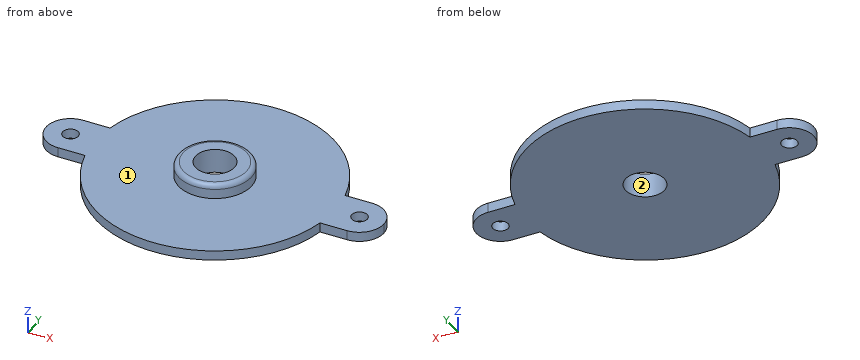
```python
from build123d import *

# Parameters (mm, degrees)
F0_R     = 1.6
F0_R_2   = 4
F1_DEPTH = 2
F2_R     = 7.5
F2_R_2   = 4
F3_DEPTH = 3
F4_R     = 1


with BuildPart() as f1:
    # F0 (on Top) → F1 (new body)
    with BuildSketch(Plane.XY):
        with BuildLine():
            ThreePointArc((-29.5, -5), (-25.964466, -3.535534), (-24.5, 0))
            ThreePointArc((-24.5, 0), (-25.964466, 3.535534), (-29.5, 5))
            ThreePointArc((-29.5, 5), (-34.5, 0), (-29.5, -5))
        make_face()
        with Locations((-29.5, 0)):
            Circle(F0_R, mode=Mode.SUBTRACT)
        with BuildLine():
            ThreePointArc((-29.5, 5), (-25.964466, 3.535534), (-24.5, 0))
            ThreePointArc((-24.5, 0), (-24.370752, 2.513259), (-23.98437, 5))
            Line((-23.98437, 5), (-29.5, 5))
        make_face()
        with BuildLine():
            ThreePointArc((-23.98437, -5), (-24.370752, -2.513259), (-24.5, 0))
            ThreePointArc((-24.5, 0), (-25.964466, -3.535534), (-29.5, -5))
            Line((-29.5, -5), (-23.98437, -5))
        make_face()
        with BuildLine():
            ThreePointArc((-23.98437, 5), (-24.370752, 2.513259), (-24.5, 0))
            ThreePointArc((-24.5, 0), (-24.370752, -2.513259), (-23.98437, -5))
            ThreePointArc((-23.98437, -5), (0, -24.5), (23.98437, -5))
            ThreePointArc((23.98437, -5), (24.370752, -2.513259), (24.5, 0))
            ThreePointArc((24.5, 0), (24.370752, 2.513259), (23.98437, 5))
            ThreePointArc((23.98437, 5), (0, 24.5), (-23.98437, 5))
        make_face()
        Circle(F0_R_2, mode=Mode.SUBTRACT)
        with BuildLine():
            ThreePointArc((29.5, 5), (25.964466, 3.535534), (24.5, 0))
            ThreePointArc((24.5, 0), (25.964466, -3.535534), (29.5, -5))
            ThreePointArc((29.5, -5), (33.035534, -3.535534), (34.5, 0))
            ThreePointArc((34.5, 0), (33.035534, 3.535534), (29.5, 5))
        make_face()
        with Locations((29.5, 0)):
            Circle(F0_R, mode=Mode.SUBTRACT)
        with BuildLine():
            ThreePointArc((24.5, 0), (24.370752, -2.513259), (23.98437, -5))
            Line((23.98437, -5), (29.5, -5))
            ThreePointArc((29.5, -5), (25.964466, -3.535534), (24.5, 0))
        make_face()
        with BuildLine():
            Line((29.5, 5), (23.98437, 5))
            ThreePointArc((23.98437, 5), (24.370752, 2.513259), (24.5, 0))
            ThreePointArc((24.5, 0), (25.964466, 3.535534), (29.5, 5))
        make_face()
    extrude(amount=F1_DEPTH)

    # F2 (on face) → F3 (join)
    with BuildSketch(Plane.XY.offset(2)):
        Circle(F2_R)
        Circle(F2_R_2, mode=Mode.SUBTRACT)
    extrude(amount=F3_DEPTH)

    # F4
    f4_edges = [f1.edges().sort_by_distance(p)[0] for p in [
        (-7.5, 0, 5),
    ]]
    fillet(f4_edges, radius=F4_R)


solid = f1.part
```
Input: part model. Units: mm. Frame: model coordinates. Face numbers are marked on the shaded views. Round coordinates to 2 decimals unless told otherwise and drop trailing zeros. Loops run counter-clockwise (first coordinate to the right, second up) from the corner with the lowest first, then second, coordinate; pieces in that order, holes last. Notation, with made-up numbers: (3, 48) - (36, 48) arc R32 ccw to (36, 75) - close; hole circle Ø5 at (24.25, -35.75). An arc over 180 degrees is marked (long way). One line per item, written item: value. Start each with the question number.
(1) Contact query for flat-ended pins moving along their axis: P1, Ø5, axis at x = 21, y = -7, coming from the -Z side; P2, Ø1, axis at x = 14.5, z = 1, coming from the -Y side; P3, Ø1.5, axis at y = -7.5, z = 1.5, coming from the +X side; P4, Ø2, axis at x = -26.5, z = 1.5, coming from the +Y side. Output: stop coordinate, or through.
(2) Section C-C, the plane x = 12.5. Return loops of the section in (y, z), plus the area to 3 significant figures.
(3) Ray query, line 1 (Y direction, x = 29.5, z = 0.65); line 2 (Z direction, x = 11, y = -12.5); line 3 (Y direction, x = 0, z = 2.5). Return the intervals inside material, ascending. Write a range as [from, to].
(4) Section B-B, the plane y = 13.5. Return loops of the section in (x, z).
(5) Draft query along Y for the marked faces 1 and 2. Return one class per face: +Y half, -Y half, draft (parallel to the pull), parting line (faces both ways), or undercut.
(6) Section A-A, the plane x = 0. Return loops of the section in (y, z), plus the area to 3 significant figures.
Results below:
1. P1: z = 0
1. P2: y = -20.11
1. P3: x = 23.55
1. P4: y = 5
2. outline: (-21.07, 0) - (21.07, 0) - (21.07, 2) - (-21.07, 2) - close
2. area: 84.3 mm^2
3. line 1: [-5, -1.6], [1.6, 5]
3. line 2: [0, 2]
3. line 3: [-7.5, -4], [4, 7.5]
4. outline: (-20.45, 0) - (20.45, 0) - (20.45, 2) - (-20.45, 2) - close
5. face 1: draft
5. face 2: undercut
6. outline: (-24.5, 0) - (-4, 0) - (-4, 5) - (-6.5, 5) arc R1 ccw to (-7.5, 4) - (-7.5, 2) - (-24.5, 2) - close; (4, 0) - (24.5, 0) - (24.5, 2) - (7.5, 2) - (7.5, 4) arc R1 ccw to (6.5, 5) - (4, 5) - close
6. area: 103 mm^2
